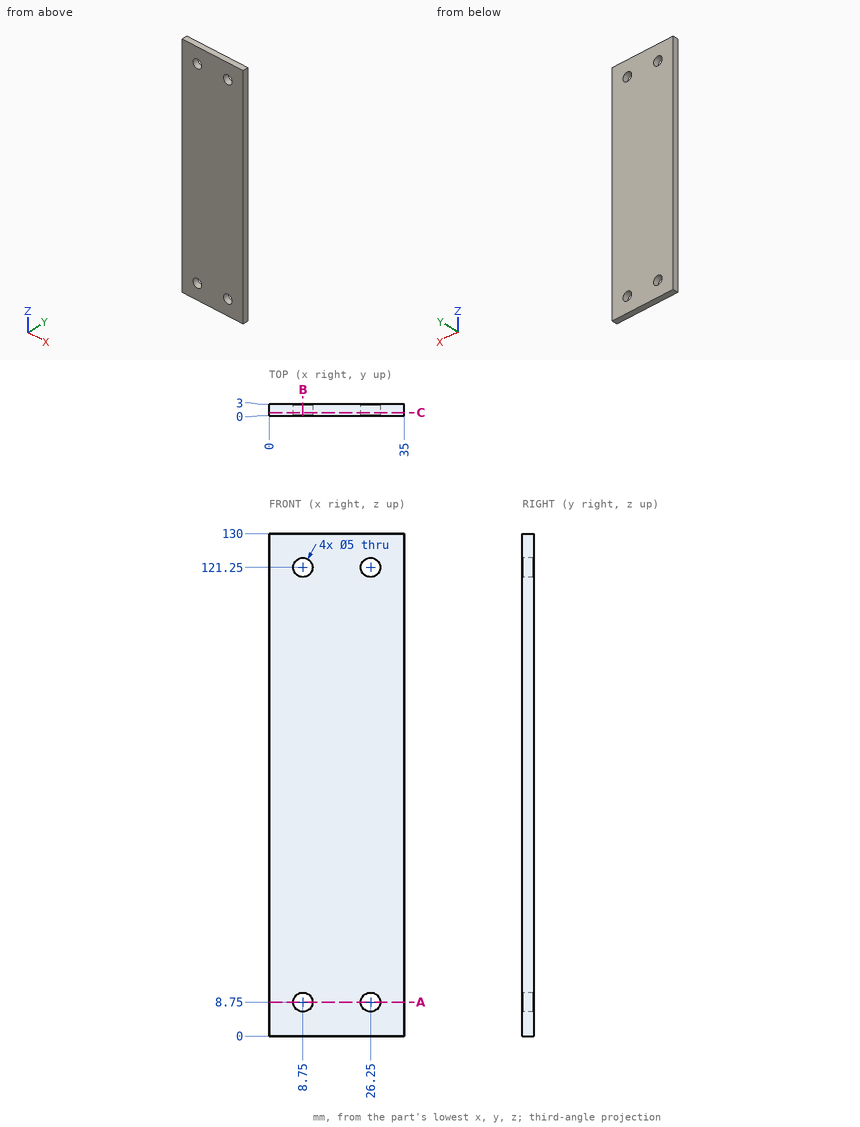
Geometry: see drawing. Coordinates: mm, zero at the bounding-box minimum. Round coordinates to 2 decimals unless told otherwise and drop trailing zeros. Write each loop counter-clockwise with the first axis right and the second up, starting at its lowest first coordinate (ties: lowest second). Pieces come first, ordered by that corner, then holes. Notation, with made-up numbers: M 75.5,73 L 104.5,73 A13 cw 104.5,91 Z; hole C 24.5,71.5 d9. An arc over 180 degrees is marked long. Answer in a Markdown table with one row per item. Add a question column.
(1) Contact query for a flat-ended pin moving along its axis: pin 1 (8 mm diameter, centred on x = 8.75, z = 121.25, fed in from -Y). Output: stop coordinate, or through.
(2) Ray query, L1, parallel to Z at x = 26, y = 1.3; L2, parallel to Z at x = 8, y = 0.7; L3, parallel to X at y = 2.4, z = 9. Return the intervals inside material, ascending.
(3) Cut plane A-A, the plane z = 8.75. Return the cut outline in (x, y), then the cut area to 3 significant figures.
(4) Cut plane B-B, the plane x = 8.75. Return the cut outline in (y, z), then the cut area to 3 significant figures.
(5) Cut plane C-C, the plane y = 0.8. Return the cut outline in (x, z), then the cut area to 3 significant figures.
Established:
| question | item | result |
|---|---|---|
| 1 | pin 1 | y = 0 |
| 2 | L1 | 0 to 6.26, 11.24 to 118.76, 123.74 to 130 |
| 2 | L2 | 0 to 6.37, 11.13 to 118.87, 123.63 to 130 |
| 2 | L3 | 0 to 6.26, 11.24 to 23.76, 28.74 to 35 |
| 3 | outline | M 0,0 L 6.25,0 L 6.25,3 L 0,3 Z; M 11.25,0 L 23.75,0 L 23.75,3 L 11.25,3 Z; M 28.75,0 L 35,0 L 35,3 L 28.75,3 Z |
| 3 | area | 75.0 mm² |
| 4 | outline | M 0,0 L 3,0 L 3,6.25 L 0,6.25 Z; M 0,11.25 L 3,11.25 L 3,118.75 L 0,118.75 Z; M 0,123.75 L 3,123.75 L 3,130 L 0,130 Z |
| 4 | area | 360 mm² |
| 5 | outline | M 0,0 L 35,0 L 35,130 L 0,130 Z; hole C 8.75,8.75 d5; hole C 8.75,121.25 d5; hole C 26.25,8.75 d5; hole C 26.25,121.25 d5 |
| 5 | area | 4,470 mm² |
